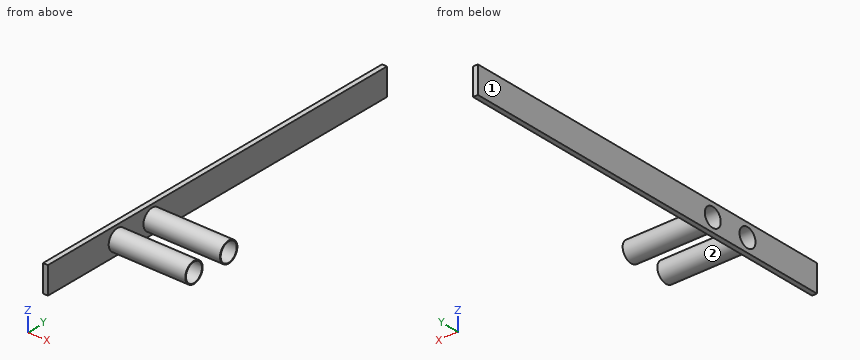
```python
from build123d import *

# Parameters (mm, degrees)
F0_W     = 976
F0_H     = 66
F0_R     = 25
F1_DEPTH = 12
F0_R_2   = 22.999999
F2_DEPTH = 200
F0_R_3   = 23
F3_DEPTH = 200


with BuildPart() as f1:
    # F0 (on Right) → F1 (new body)
    with BuildSketch(Plane.YZ):
        with Locations((488, 33)):
            Rectangle(F0_W, F0_H)
        with Locations((200, 33)):
            Circle(F0_R, mode=Mode.SUBTRACT)
        with Locations((300, 33)):
            Circle(F0_R, mode=Mode.SUBTRACT)
    extrude(amount=F1_DEPTH)

    # F0 (on Right) → F2 (join)
    with BuildSketch(Plane.YZ):
        with Locations((200, 33)):
            Circle(F0_R)
        with Locations((200, 33)):
            Circle(F0_R_2, mode=Mode.SUBTRACT)
    extrude(amount=F2_DEPTH)

    # F0 (on Right) → F3 (join)
    with BuildSketch(Plane.YZ):
        with Locations((300, 33)):
            Circle(F0_R)
        with Locations((300, 33)):
            Circle(F0_R_3, mode=Mode.SUBTRACT)
    extrude(amount=F3_DEPTH)


solid = f1.part
```
The listing builds one solid part. Answer for the finished solid, in the listing's coordinates (mm). Face numbers are marked on the shaded views. Give positions to 0.01 mm unless a question says otherwise; leave off trailing zeros. Loops run counter-clockwise (first coordinate to the right, second up) from the corner with the lowest first, then second, coordinate; pieces in that order, holes last. Notation, with made-up numbers: (6, -11.75) - (50, -11.75) arc R24 ccw to (50, 7.25) - close; hole circle Ø10 at (52, 46). An arc over 180 degrees is marked (long way). Answer as CSV lines item,"result". Start each with the question number.
Item 1: A cutting plane is placed at D-D on y = 796. Determine the outline of the cut face in (x, z).
Item 2: Each of these flat-tipped pins is pushed along its axis until it touches: pin 1 (5 mm diameter, centred on x = 69, z = 35.5, fed in from +Y); pin 2 (6 mm diameter, centred on y = 699.5, z = 59, fed in from +X); pin 3 (12 mm diameter, centred on y = 128, z = 48.5, fed in from -X); pin 4 (8 mm diameter, centred on x = 28.5, z = 34.5, fed in from -Y). Where does it stop, or does it pass through?
Item 3: Find the intervals of material crossed by line 1 (Z direction, x = 59, y = 200); line 2 (Y direction, x = 129.5, z = 48.5); line 3 (Y direction, x = 145.5, z = 36.5), in increasing order. Write a range as from..to.
Item 4: The mould has two halves that part along Y. Classify the marked faces 1 and 2: +Y half, -Y half, draft (parallel to the pull), parting line (faces both ways), or undercut.
Item 5: A cutting plane is placed at C-C on x = 135. Determine the outline of the cut face in (y, z), then the cut area to 3 significant figures.
Item 6: A cutting plane is placed at B-B on z = 33. Determine the outline of the cut face in (x, y), then the cut area to 3 significant figures.
Item 7: A cutting plane is placed at A-A on y = 300. Determine the outline of the cut face in (x, z), then the cut area to 3 significant figures.
Found:
1,outline,"(0, 0) - (12, 0) - (12, 66) - (0, 66) - close"
2,pin 1,"stops at y = 325"
2,pin 2,"stops at x = 12"
2,pin 3,"stops at x = 0"
2,pin 4,"stops at y = 175"
3,line 1,"z = 8..10, 56..58"
3,line 2,"y = 180.38..183.01, 216.99..219.62, 280.38..283.01, 316.99..319.62"
3,line 3,"y = 175.25..177.27, 222.73..224.75, 275.25..277.27, 322.73..324.75"
4,face 1,"draft"
4,face 2,"undercut"
5,outline,"circle Ø50 at (200, 33); circle Ø50 at (300, 33); hole circle Ø46 at (200, 33); hole circle Ø46 at (300, 33)"
5,area,"603 mm^2"
6,outline,"(0, 0) - (12, 0) - (12, 175) - (200, 175) - (200, 177) - (0, 177) - close; (0, 223) - (200, 223) - (200, 225) - (12, 225) - (12, 275) - (200, 275) - (200, 277) - (0, 277) - close; (0, 323) - (200, 323) - (200, 325) - (12, 325) - (12, 976) - (0, 976) - close"
6,area,"12,100 mm^2"
7,outline,"(0, 0) - (12, 0) - (12, 8) - (200, 8) - (200, 10) - (0, 10) - close; (0, 56) - (200, 56) - (200, 58) - (12, 58) - (12, 66) - (0, 66) - close"
7,area,"992 mm^2"
